Geometry check sheet. Reference: drawing and pictorial views, mm from the part's lowest x, y, z. A direction names the side the tool comes from. Give positions to 0.01 mm unless a question says otherwise; leave off trailing zeros. Order: outer loops, then holes, each group sorted by start corner. A loop starts at its lowest first (then second) coordinate and runs counter-clockwise, first axis right, second up.
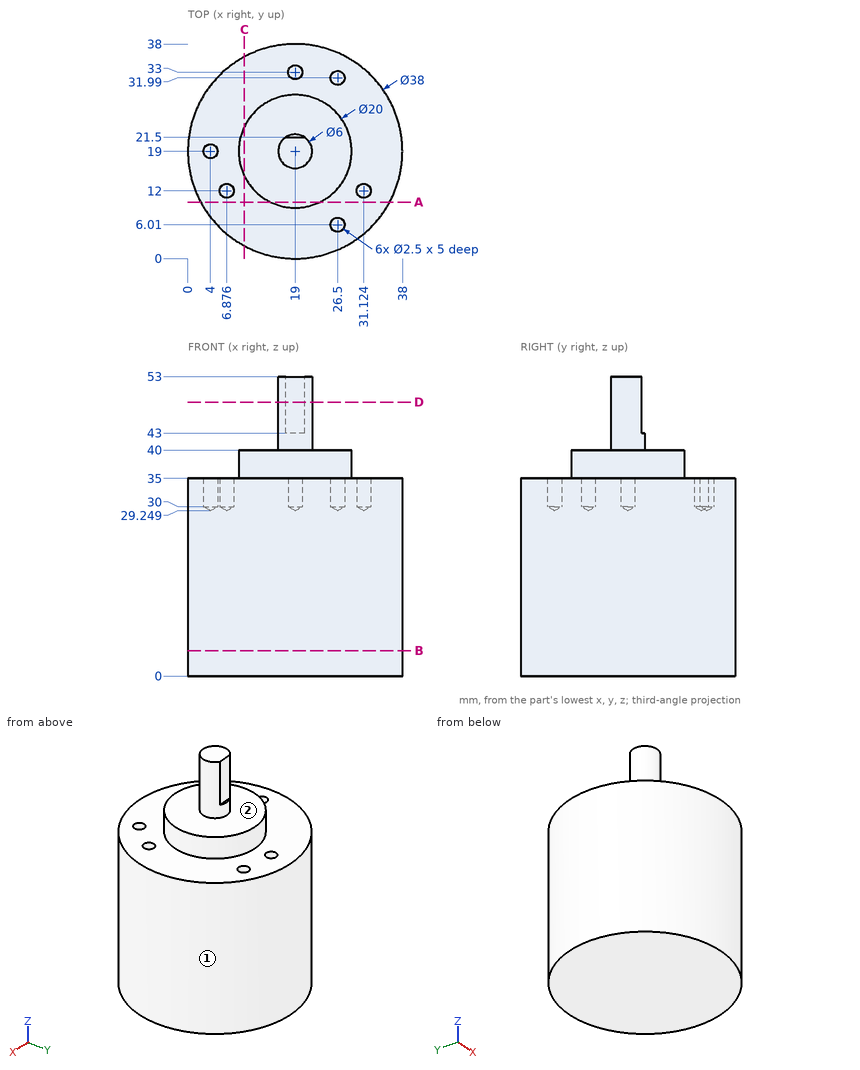
(1) Cross-section at B-B on z = 4.5. Enter the section's corners in (x, y), then the cut area to 3 significant figures.
Response values:
outline: circle Ø38 at (19, 19)
area: 1,130 mm2
(2) Material ranges on L1, parallel to Y at x = 26.5, z = 31.5; L2, parallel to X at y = 12, z = 31 (1 decimal); L3, parallel to Z at x = 18.5, y = 11.5, recorded low to high.
Response values:
L1: y = 1.54 to 4.76, 7.26 to 30.74, 33.24 to 36.46
L2: x = 1.3 to 5.6, 8.1 to 29.9, 32.4 to 36.7
L3: z = 0 to 40
(3) Cross-section at D-D on z = 48.5. Enter the section's corners in (x, y).
Response values:
outline: (17.34, 21.5) arc R3 ccw (long way) to (20.66, 21.5) - close
(4) Set-up check for the marked faces 1 and 2: record each of +Z, -Z, +X, -X, +Y, -Y from which the full face is reachable in a straight line by a thin tool's end or side.
Response values:
face 1: +Z, -Z
face 2: +Z
(5) Gauge pin test, flat ends, axial feed: pin 1 Ø1.5 at (x, y) = (25.5, 11.5) entering from +Z; pin 2 Ø1 at (y, z) = (16.5, 45.5) entering from +X (1 decimal); pin 3 Ø1.5 at (x, y) = (19, 33) entering from +Z; pin 4 Ø5 at (x, z) = (25.5, 44) entering from +Y. Record the tip position at first contact, or that the pin passes through.
Response values:
pin 1: stops at z = 40
pin 2: stops at x = 21.2
pin 3: stops at z = 29.7
pin 4: passes through
(6) Cross-section at A-A on y = 10. Enter the section's corners in (x, z).
Response values:
outline: (2.27, 0) - (35.73, 0) - (35.73, 35) - (23.36, 35) - (23.36, 40) - (14.64, 40) - (14.64, 35) - (2.27, 35) - close
